For this review, use the dimensioned drawing (mm, ordinates from the lowest corner) and the shaded views. A direction names the side the tool comes from. Round coordinates to 2 decimals unless told otherwise and drop trailing zeros. Order: outer loops, then holes, each group sorted by start corner. A loop starts at its lowest first (then second) coordinate and runs counter-clockwise, first axis right, second up. Notation, with made-up numbers: (-17.75, 76) - (29.25, 76) arc R18 cw to (29.25, 81) - close; hole circle Ø9 at (8.25, -40). An arc over 180 degrees is marked (long way). Write each question's results on one line, items separated by ' | '. Start each with the question number.
(1) Take a section at A-A, the plane y = 9.5. Give the boundary of the cut face in (x, z), plus the area to 4 significant figures.
(2) For L1, parallel to Z at x = 10.25, y = 2.25; L2, parallel to Z at x = 17.5, y = 7.75; L3, parallel to Y at x = 9.25, z = 10.5, list the stretches that pass through material, from the lowest coordinate up. Write a range as from..to.
(3) Take a section at C-C, the plane z = 14.25. Give the boundary of the cut face in (x, y).
(4) For the marked faces 1 and 2, list the 3-axis set-ups (+Z, -Z, +X, -X, +Y, -Y) from which the entire face can be reached by the end or side of a thin tool; tool diameter is ignored.
(5) Insertion check: pin 1 Ø6 at (y, z) = (7, 20) entering from -X. The pin has a flat end and moves straight along its axis. Give the tip position at first contact, or say it passes through.
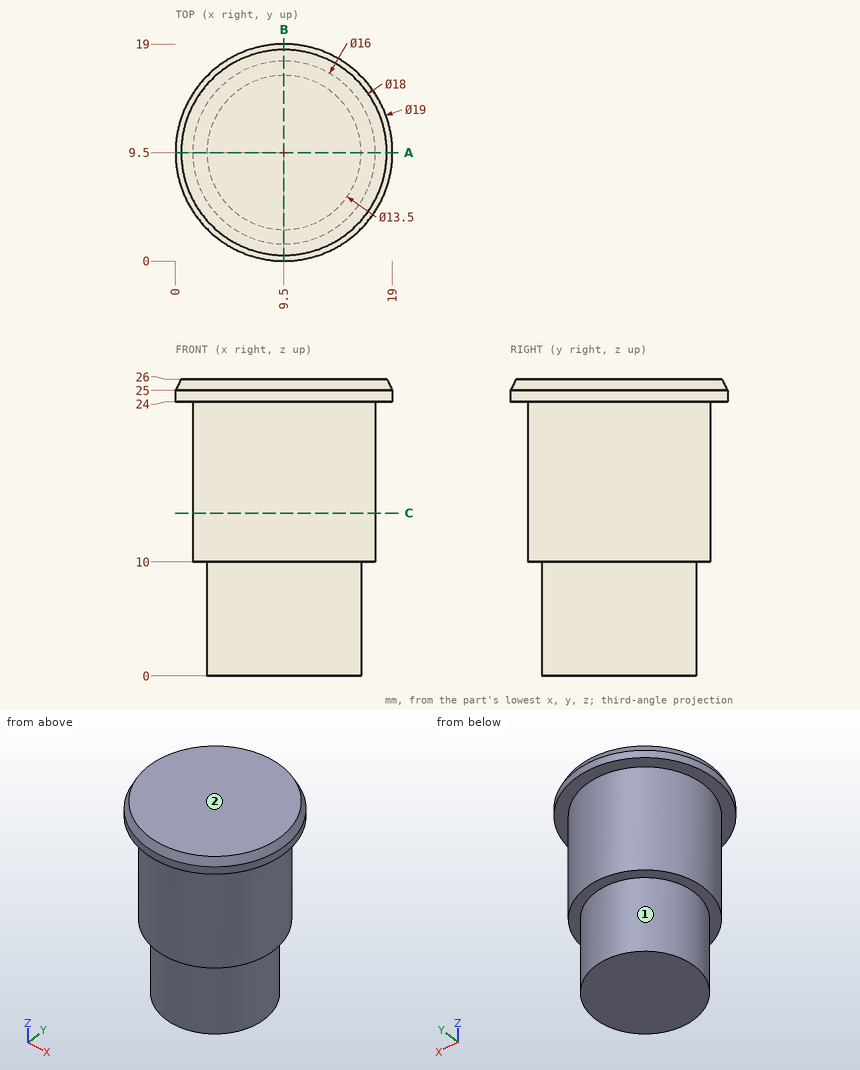
Results below:
1) outline: (0, 24) - (1.5, 24) - (1.5, 10) - (2.75, 10) - (2.75, 0) - (16.25, 0) - (16.25, 10) - (17.5, 10) - (17.5, 24) - (19, 24) - (19, 25) - (18.5, 26) - (0.5, 26) - (0, 25) - close | area: 396.5 mm^2
2) L1: z = 10..26 | L2: z = 24..26 | L3: y = 1.5..17.5
3) outline: circle Ø16 at (9.5, 9.5)
4) face 1: -Z | face 2: +Z, +X, -X, +Y, -Y
5) pin 1: stops at x = 1.5
